from build123d import *

# Parameters (mm, degrees)
SKETCH1_R                = 3.6
SKETCH1_R_2              = 2.5
MAIN_BOSS_DEPTH          = 2.5
SKETCH2_R                = 2
SMALL_HOLE_EXTRUDE_DEPTH = 1.5
SKETCH3_R                = 1.5
SMALL_HOLE_DEPTH         = 58.412977627
SKETCH4_R                = 2
LONG_HOLE_EXTRUDE_DEPTH  = 4.5
SKETCH5_R                = 1.5
LONG_HOLE_DEPTH          = 58.900777197
SIDE_BOSS_DEPTH          = 1.5


with BuildPart() as part:
    # Sketch1 → main boss (new body)
    with BuildSketch(Plane(origin=(0, 0, 0), x_dir=(1, 0, 0), z_dir=(0, 1, 0))):
        with BuildLine():
            Line((32, 0), (12, 0))
            Line((12, 0), (12, -4.5))
            ThreePointArc((12, -4.5), (0, -16.5), (-12, -4.5))
            Line((-12, -4.5), (-12, 0))
            Line((-12, 0), (-32, 0))
            Line((-32, 0), (-32, 37.5))
            ThreePointArc((-32, 37.5), (-29.071067812, 44.571067812), (-22, 47.5))
            Line((-22, 47.5), (22, 47.5))
            ThreePointArc((22, 47.5), (29.071067812, 44.571067812), (32, 37.5))
            Line((32, 37.5), (32, 0))
        make_face()
        with Locations(Location((0, -4.6, 0), (0, 0, 270))):
            Circle(SKETCH1_R, mode=Mode.SUBTRACT)
        with Locations(Location((20, 35.6, 0), (0, 0, 270))):
            Circle(SKETCH1_R_2, mode=Mode.SUBTRACT)
        with Locations(Location((-20, 35.6, 0), (0, 0, 270))):
            Circle(SKETCH1_R_2, mode=Mode.SUBTRACT)
    extrude(amount=MAIN_BOSS_DEPTH)

    # Sketch2 → small hole extrude (add)
    with BuildSketch(Plane(origin=(0, 2.5, 0), x_dir=(1, 0, 0), z_dir=(0, 1, 0))):
        with Locations(Location((1.5, 33.15, 0), (0, 0, 270))):
            Circle(SKETCH2_R)
        with Locations(Location((19, 14.25, 0), (0, 0, 270))):
            Circle(SKETCH2_R)
    extrude(amount=SMALL_HOLE_EXTRUDE_DEPTH)

    # Sketch3 → small hole (cut, through all)
    with BuildSketch(Plane(origin=(0, 4, 0), x_dir=(1, 0, 0), z_dir=(0, 1, 0))):
        with Locations(Location((1.5, 33.15, 0), (0, 0, 270))):
            Circle(SKETCH3_R)
        with Locations(Location((19, 14.25, 0), (0, 0, 270))):
            Circle(SKETCH3_R)
    extrude(amount=-SMALL_HOLE_DEPTH, mode=Mode.SUBTRACT)

    # Sketch4 → long hole extrude (add)
    with BuildSketch(Plane.XZ):
        with Locations(Location((-23.5, -23.05, 0), (0, 0, 90))):
            Circle(SKETCH4_R)
        with Locations(Location((-9.5, -23.05, 0), (0, 0, 90))):
            Circle(SKETCH4_R)
    extrude(amount=LONG_HOLE_EXTRUDE_DEPTH)

    # Sketch5 → long hole (cut, through all)
    with BuildSketch(Plane.XZ.offset(4.5)):
        with Locations(Location((-23.5, -23.05, 0), (0, 0, 270))):
            Circle(SKETCH5_R)
        with Locations(Location((-9.5, -23.05, 0), (0, 0, 270))):
            Circle(SKETCH5_R)
    extrude(amount=-LONG_HOLE_DEPTH, mode=Mode.SUBTRACT)

    # Sketch6 → side boss (add)
    with BuildSketch(Plane.XY):
        with BuildLine():
            Line((-32, 0), (-32, 15))
            ThreePointArc((-32, 15), (-31.414213562, 16.414213562), (-30, 17))
            Line((-30, 17), (-21.5, 17))
            Line((-21.5, 17), (-21.5, 6))
            Line((-21.5, 6), (-20, 6))
            Line((-20, 6), (-20, 17))
            Line((-20, 17), (-17, 17))
            ThreePointArc((-17, 17), (-15.585786438, 16.414213562), (-15, 15))
            Line((-15, 15), (-15, 0))
            Line((-15, 0), (-32, 0))
        make_face()
    side_boss = extrude(amount=-SIDE_BOSS_DEPTH)

    # Mirror1: side boss across plane
    add(side_boss.mirror(Plane(origin=(0, 0, 0), x_dir=(0, 0, 1), z_dir=(1, 0, 0))))


solid = part.part
Verification items for the finished model (mm, model axes). A direction names the side the tool comes from. Round coordinates to 2 decimals unless told otherwise and drop trailing zeros. Order: outer loops, then holes, each group sorted by start corner. A loop starts at its lowest first (then second) coordinate and runs counter-clockwise, first axis right, second up.
1. Thickness scan on L1, parallel to X at y = 1, z = -35.6; L2, parallel to X at y = -0.5, z = -23.05; L3, parallel to X at y = 1.2, z = -14.25. Record the ranges inside material, lowest first.
Final values:
L1: x = -32 to -22.5, -17.5 to 17.5, 22.5 to 32
L2: x = -25.5 to -25, -22 to -21.5, -11.5 to -11, -8 to -7.5
L3: x = -32 to 17.5, 20.5 to 32
2. Section check A-A on y = 7.5. Record the cut outline in (x, z), then the cut area to 3 significant figures.
Final values:
outline: (-32, -1.5) - (-21.5, -1.5) - (-21.5, 0) - (-32, 0) - close; (-20, -1.5) - (-15, -1.5) - (-15, 0) - (-20, 0) - close; (15, -1.5) - (20, -1.5) - (20, 0) - (15, 0) - close; (21.5, -1.5) - (32, -1.5) - (32, 0) - (21.5, 0) - close
area: 46.5 mm2
3. Section check C-C on y = 1.25. Record the cut outline in (x, z), then the cut area to 3 significant figures.
Final values:
outline: (-32, -37.5) arc R10 ccw to (-22, -47.5) - (22, -47.5) arc R10 ccw to (32, -37.5) - (32, 0) - (12, 0) - (12, 4.5) arc R12 ccw to (-12, 4.5) - (-12, 0) - (-32, 0) - close; hole circle Ø3 at (-23.5, -23.05); hole circle Ø5 at (-20, -35.6); hole circle Ø3 at (-9.5, -23.05); hole circle Ø7.2 at (0, 4.6); hole circle Ø3 at (1.5, -33.15); hole circle Ø5 at (20, -35.6); hole circle Ø3 at (19, -14.25)
area: 3,220 mm2
4. Section check D-D on x = 1.5. Record the cut outline in (y, z), then the cut area to 3 significant figures.
Final values:
outline: (0, -47.5) - (2.5, -47.5) - (2.5, -35.15) - (4, -35.15) - (4, -34.65) - (0, -34.65) - close; (0, -31.65) - (4, -31.65) - (4, -31.15) - (2.5, -31.15) - (2.5, 1.33) - (0, 1.33) - close; (0, 7.87) - (2.5, 7.87) - (2.5, 16.41) - (0, 16.41) - close
area: 137 mm2
5. Go/stop test with flat-tipped pins: P1, Ø3, axis at y = 1.5, z = 2.5, coming from the -X side; P2, Ø3.5, axis at x = 19, z = -14.25, coming from the -Y side; P3, Ø12, axis at x = 15.5, y = 9, coming from the -Z side. Record where each tip stops, or that it passes through.
Final values:
P1: stops at x = -12
P2: stops at y = 0
P3: stops at z = -16.24
6. Access from +Z, -Z, +X, -X, +Y, -Y to the whole of each face (thin tool, end or side, straight path). Record for faces 1 (the flat face through (19, 4, -16)), 2 (the cylindrical face through (-22.734, -2.218, -21.203)), 3 (the flat face through (-12, 1, 2)), 4 (the flat face through (21.5, 12, -1)), 5 (the cylindrical face through (0, 1, 1)).
Final values:
face 1: -Z, +X, -X, +Y
face 2: -Y
face 3: +Z, -X, +Y, -Y
face 4: +Z, -Z, +Y
face 5: +Y, -Y
7. Section check B-B on z = -23.05. Record the cut outline in (x, y).
Final values:
outline: (-32, 0) - (-25.5, 0) - (-25.5, -4.5) - (-25, -4.5) - (-25, 2.5) - (-32, 2.5) - close; (-22, -4.5) - (-21.5, -4.5) - (-21.5, 0) - (-11.5, 0) - (-11.5, -4.5) - (-11, -4.5) - (-11, 2.5) - (-22, 2.5) - close; (-8, -4.5) - (-7.5, -4.5) - (-7.5, 0) - (32, 0) - (32, 2.5) - (-8, 2.5) - close
8. Release check for a two-part mould opening along X. For faces 6 (the flat face through (21, 6, -1)), 7 (the flat face through (23, 10, -1.5)), 8 (the flat face through (12, 1, 2)) record: +X half, -X half, draft (parallel to the pull), parting line (faces both ways), or undercut.
Final values:
face 6: undercut
face 7: draft
face 8: +X half
